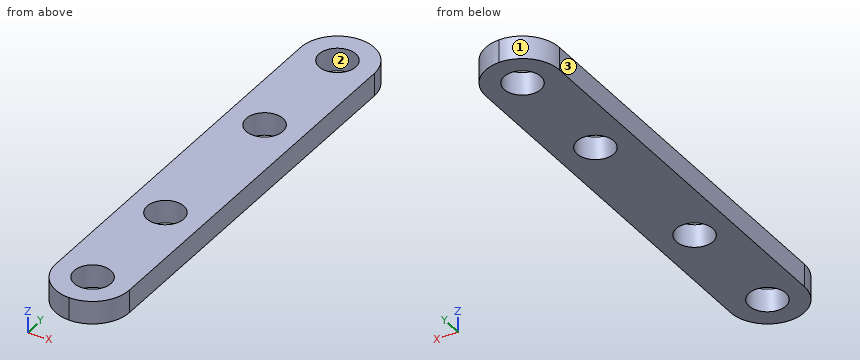
```python
from build123d import *

# Parameters (mm, degrees)
F0_W     = 16
F0_H     = 100
F1_DEPTH = 5
F2_R     = 7.99999
F4_D     = 8


# Not quite as in the source:
# - a fillet or chamfer is up to 0.001 mm smaller than in the source, because OpenCascade refuses the exact size


with BuildPart() as f1:
    # F0 (on Top) → F1 (new body)
    with BuildSketch(Plane.XY):
        with Locations((8, 50)):
            Rectangle(F0_W, F0_H)
    extrude(amount=F1_DEPTH)

    # F2 (radius 8 in the source; OpenCascade refuses exactly that, so slightly less here)
    f2_edges = [f1.edges().sort_by_distance(p)[0] for p in [
        (16, 0, 2.5),
        (0, 0, 2.5),
        (16, 100, 2.5),
        (0, 100, 2.5),
    ]]
    fillet(f2_edges, radius=F2_R)

    # F4 (through all)
    with Locations(Plane.XY.offset(5)):
        with Locations((8, 92), (8, 67), (8, 33), (8, 8)):
            Hole(F4_D / 2)


solid = f1.part
```
Build history of the part. All positions in model axes, mm. Face numbers are marked on the shaded views. Coordinates: 2 decimals unless noted, no trailing zeros. Order: outer loops, then holes, each group sorted by start corner. A loop starts at its lowest first (then second) coordinate and runs counter-clockwise, first axis right, second up. Notation, with made-up numbers: (-8.5, 14) -> (11.5, 14) arc R17 cw to (11.5, 19) -> close; hole circle Ø6 at (73, -7.75). An arc over 180 degrees is marked (long way). Answer in a Markdown table with one row per item. Add a question column.
Q1. Band-saw the part on D-D, the plane x = 9.25. List the corners of the cut face in (y, z), then the cut area to 3 significant figures.
Q2. Mould opens along Y. For the marked faces 1, 2 and 3 say: +Y half, -Y half, draft (parallel to the pull), parting line (faces both ways), or undercut.
Q3. Band-saw the part on C-C, the plane z = 2.35. Give the number of separate pieces and of enclosed holes in the cut face, then the cut area to 3 significant figures.
Q4. Wall check: line 1 along Y through (x, z) = (8, 3.7); line 2 along Y through (x, z) = (4.5, 3.15); line 3 along Y through (x, z) = (14.5, 3.5). Give the ranges that are in metal, low to high. Write a range as [from, to].
Q5. Band-saw the part on B-B, the plane x = 5. List the corners of the cut face in (y, z), then the cut area to 3 significant figures.
Q6. Band-saw the part on A-A, the plane y = 33. List the corners of the cut face in (x, z).
Answers follow:
| question | item | result |
|---|---|---|
| 1 | outline | (0.1, 0) -> (4.2, 0) -> (4.2, 5) -> (0.1, 5) -> close; (11.8, 0) -> (29.2, 0) -> (29.2, 5) -> (11.8, 5) -> close; (36.8, 0) -> (63.2, 0) -> (63.2, 5) -> (36.8, 5) -> close; (70.8, 0) -> (88.2, 0) -> (88.2, 5) -> (70.8, 5) -> close; (95.8, 0) -> (99.9, 0) -> (99.9, 5) -> (95.8, 5) -> close |
| 1 | area | 347 mm^2 |
| 2 | face 1 | +Y half |
| 2 | face 2 | undercut |
| 2 | face 3 | draft |
| 3 | separate pieces | 1 |
| 3 | enclosed holes | 4 |
| 3 | area | 1,340 mm^2 |
| 4 | line 1 | [0, 4], [12, 29], [37, 63], [71, 88], [96, 100] |
| 4 | line 2 | [0.81, 6.06], [9.94, 31.06], [34.94, 65.06], [68.94, 90.06], [93.94, 99.19] |
| 4 | line 3 | [3.34, 96.66] |
| 5 | outline | (0.58, 0) -> (5.35, 0) -> (5.35, 5) -> (0.58, 5) -> close; (10.65, 0) -> (30.35, 0) -> (30.35, 5) -> (10.65, 5) -> close; (35.65, 0) -> (64.35, 0) -> (64.35, 5) -> (35.65, 5) -> close; (69.65, 0) -> (89.35, 0) -> (89.35, 5) -> (69.65, 5) -> close; (94.65, 0) -> (99.42, 0) -> (99.42, 5) -> (94.65, 5) -> close |
| 5 | area | 388 mm^2 |
| 6 | outline | (0, 0) -> (4, 0) -> (4, 5) -> (0, 5) -> close; (12, 0) -> (16, 0) -> (16, 5) -> (12, 5) -> close |
